from build123d import *

# Parameters (mm, degrees)
SKETCH1_R           = 20
SKETCH1_R_2         = 15
BOSS_EXTRUDE1_DEPTH = 200
BOSS_EXTRUDE5_START = 5
BOSS_EXTRUDE5_DEPTH = 8
BOSS_EXTRUDE6_START = -5
BOSS_EXTRUDE6_DEPTH = 8
BOSS_EXTRUDE7_START = -8
SKETCH7_R           = 3.5
BOSS_EXTRUDE7_DEPTH = 10


with BuildPart() as part:
    # Sketch1 → Boss-Extrude1 (new body, symmetric)
    with BuildSketch(Plane.XY):
        Circle(SKETCH1_R)
        Circle(SKETCH1_R_2, mode=Mode.SUBTRACT)
    extrude(amount=BOSS_EXTRUDE1_DEPTH, both=True)

    # Sketch6 → Boss-Extrude5 (add)
    with BuildSketch(Plane(origin=(0, 0, 0), x_dir=(1, 0, 0), z_dir=(0, 1, 0)).offset(BOSS_EXTRUDE5_START)):
        with BuildLine():
            Line((-20, 200), (20, 200))
            Line((20, 200), (20, 215))
            ThreePointArc((20, 215), (0, 235), (-20, 215))
            Line((-20, 215), (-20, 200))
        make_face()
    extrude(amount=BOSS_EXTRUDE5_DEPTH)

    # Sketch6_2 → Boss-Extrude6 (add)
    with BuildSketch(Plane(origin=(0, 0, 0), x_dir=(1, 0, 0), z_dir=(0, 1, 0)).offset(BOSS_EXTRUDE6_START)):
        with BuildLine():
            Line((-20, 200), (20, 200))
            Line((20, 200), (20, 215))
            ThreePointArc((20, 215), (0, 235), (-20, 215))
            Line((-20, 215), (-20, 200))
        make_face()
    extrude(amount=-BOSS_EXTRUDE6_DEPTH)

    # Sketch7 → Boss-Extrude7 (add)
    with BuildSketch(Plane.XZ.offset(13).offset(BOSS_EXTRUDE7_START)):
        with Locations((0, -215)):
            Circle(SKETCH7_R)
    extrude(amount=-BOSS_EXTRUDE7_DEPTH)


solid = part.part
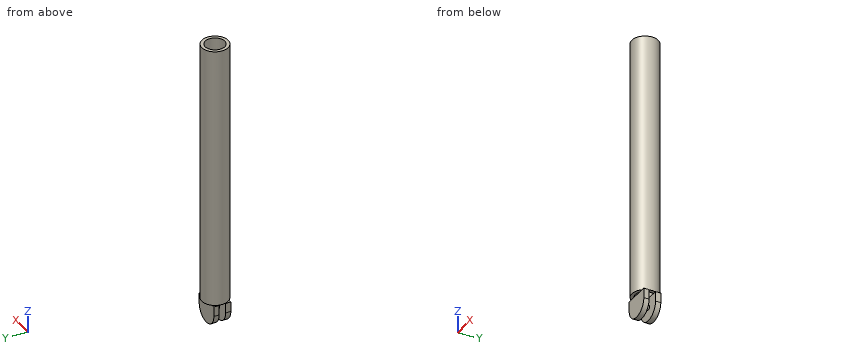
Geometry check sheet. Reference: the model listing, model coordinates, mm. Round coordinates to 2 decimals unless told otherwise and drop trailing zeros. Order: outer loops, then holes, each group sorted by start corner. A loop starts at its lowest first (then second) coordinate and runs counter-clockwise, first axis right, second up. Notation, with made-up numbers: (5.25, -0.75) - (64.25, -0.75) arc R16 cw to (64.25, 24.25) - close; hole circle Ø3 at (22.5, -15.75). An arc over 180 degrees is marked (long way). One line per question, with ' | ' between items. Start each with the question number.
(1) Depth check by flat-ended pin: pin 1 Ø1.5 at (y, z) = (-13, -41.5) entering from -X; pin 2 Ø2.5 at (x, y) = (0.5, -9.5) entering from +Z; pin 3 Ø1.5 at (x, z) = (3.5, 123.5) entering from +Y. Enter the tip coordinate at first touch or a pass-through.
(2) Thickness scan on L1, parallel to X at y = 0, z = 35; L2, parallel to X at y = 6, z = -173.5. Record the ranges inside material, lowest first. Write a range as [from, to].
(3) Sectioned sample at B-B on z = 69.5. Record the cut outline in (x, y).
(4) Sectioned sample at A-A on y = 0. Record the cut outline in (x, z), and give its area (3 significant figures).
Conclusion:
1) pin 1: stops at x = -15.81 | pin 2: stops at z = -200 | pin 3: stops at y = 19.81
2) L1: x = [-20, -15], [15, 20] | L2: x = [-19.08, -13.75], [13.75, 19.08]
3) outline: circle Ø40 at (0, 0); hole circle Ø30 at (0, 0)
4) outline: (-20, -200) - (-15, -200) - (-15, 200) - (-20, 200) - close; circle Ø7 at (0, -215); (15, -200) - (20, -200) - (20, 200) - (15, 200) - close | area: 4,040 mm2
